```python
from build123d import *

# Parameters (mm, degrees)
SKETCH1_R           = 15.875
BOSS_EXTRUDE1_DEPTH = 76.2
SKETCH2_R           = 22.225
BOSS_EXTRUDE2_DEPTH = 152.4
SKETCH3_R           = 15.875
BOSS_EXTRUDE3_DEPTH = 76.2
FILLET1_R           = 0.254
FILLET2_R           = 0.254
FILLET3_R           = 0.254
FILLET4_R           = 0.254


with BuildPart() as part:
    # Sketch1 → Boss-Extrude1 (new body)
    with BuildSketch(Plane(origin=(0, 0, 0), x_dir=(1, 0, 0), z_dir=(0, 1, 0))):
        with Locations(Location((0, 0, 0), (0, 0, 90))):
            Circle(SKETCH1_R)
    extrude(amount=BOSS_EXTRUDE1_DEPTH)

    # Sketch2 → Boss-Extrude2 (add)
    with BuildSketch(Plane(origin=(0, 76.2, 0), x_dir=(1, 0, 0), z_dir=(0, 1, 0))):
        with Locations(Location((0, 0, 0), (0, 0, 90))):
            Circle(SKETCH2_R)
    extrude(amount=BOSS_EXTRUDE2_DEPTH)

    # Sketch3 → Boss-Extrude3 (add)
    with BuildSketch(Plane(origin=(0, 228.6, 0), x_dir=(1, 0, 0), z_dir=(0, 1, 0))):
        with Locations(Location((0, 0, 0), (0, 0, 90))):
            Circle(SKETCH3_R)
    extrude(amount=BOSS_EXTRUDE3_DEPTH)

    # Fillet1
    fillet1_edges = [part.edges().sort_by_distance(p)[0] for p in [
        (0, 76.2, 15.875),
    ]]
    fillet(fillet1_edges, radius=FILLET1_R)

    # Fillet2
    fillet2_edges = [part.edges().sort_by_distance(p)[0] for p in [
        (0, 228.6, 15.875),
    ]]
    fillet(fillet2_edges, radius=FILLET2_R)

    # Fillet3
    fillet3_edges = [part.edges().sort_by_distance(p)[0] for p in [
        (0, 228.6, 22.225),
    ]]
    fillet(fillet3_edges, radius=FILLET3_R)

    # Fillet4
    fillet4_edges = [part.edges().sort_by_distance(p)[0] for p in [
        (0, 76.2, 22.225),
    ]]
    fillet(fillet4_edges, radius=FILLET4_R)


solid = part.part
```
For this review, take the finished solid that the model builds, in its own axes (mm). A direction names the side the tool comes from. Coordinates: 2 decimals unless noted, no trailing zeros. Write each loop counter-clockwise with the first axis right and the second up, starting at its lowest first coordinate (ties: lowest second). Pieces come first, ordered by that corner, then holes. Notation, with made-up numbers: (-28, -6.5) - (-18, -6.5) arc R22 ccw to (-18, 9.5) - close; hole circle Ø2 at (36.5, 55). An arc over 180 degrees is marked (long way). Answer in a Markdown table with one row per item. Add a question column.
Q1. For probe 1 along Y at (x, z) = (-19, 1.5); probe 2 along Z at (x, y) = (-1.5, 173); probe 3 along Z at (x, y) = (19, 195), list the stretches that pass through material, from the lowest coordinate up.
Q2. We need section A-A, the plane z = 0. State the section outline as (x, y) points (3 decimals).
Q3. We need section D-D, the plane y = 133.5. State the section outline as (x, z) points (3 decimals), and give its area (3 significant figures).
Q4. Tool access review of faces 1 (the cylindrical face through (-18.74, 151.34, -11.95)), 2 (the cylindrical face through (15.497, 266.295, 3.441)), 3 (the cylindrical face through (15.497, 37.441, 3.441)): name each direction out of +Z, -Z, +X, -X, +Y, -Y from which nothing blocks a thin tool from reaching the whole face with its end or side.
Q5. We need section B-B, the plane x = 0. State the section outline as (y, z) points (3 decimals), and give its area (3 significant figures).
Q6. We need section C-C, the plane y = 233.5. State the section outline as (x, z) points (3 decimals), and give its area (3 significant figures).
Q7. For P1, Ø10, axis at x = 5.5, y = 123.5, coming from the -Z side; P2, Ø2, axis at y = 71, z = 2, coming from the +X side; P3, Ø3, axis at x = 6, y = 178.5, coming from the +Z side, all flat-tipped, find the tip position at first contact; note any pin that passes through.
Answer list:
| question | item | result |
|---|---|---|
| 1 | probe 1 | y = 76.2 to 228.6 |
| 1 | probe 2 | z = -22.17 to 22.17 |
| 1 | probe 3 | z = -11.53 to 11.53 |
| 2 | outline | (-22.225, 76.454) arc R0.254 ccw to (-21.971, 76.2) - (-16.129, 76.2) arc R0.254 cw to (-15.875, 75.946) - (-15.875, 0) - (15.875, 0) - (15.875, 75.946) arc R0.254 cw to (16.129, 76.2) - (21.971, 76.2) arc R0.254 ccw to (22.225, 76.454) - (22.225, 228.346) arc R0.254 ccw to (21.971, 228.6) - (16.129, 228.6) arc R0.254 cw to (15.875, 228.854) - (15.875, 304.8) - (-15.875, 304.8) - (-15.875, 228.854) arc R0.254 cw to (-16.129, 228.6) - (-21.971, 228.6) arc R0.254 ccw to (-22.225, 228.346) - close |
| 3 | outline | circle Ø44.45 at (0, 0) |
| 3 | area | 1,550 mm2 |
| 4 | face 1 | +Y, -Y |
| 4 | face 2 | +Y |
| 4 | face 3 | -Y |
| 5 | outline | (0, -15.875) - (75.946, -15.875) arc R0.254 cw to (76.2, -16.129) - (76.2, -21.971) arc R0.254 ccw to (76.454, -22.225) - (228.346, -22.225) arc R0.254 ccw to (228.6, -21.971) - (228.6, -16.129) arc R0.254 cw to (228.854, -15.875) - (304.8, -15.875) - (304.8, 15.875) - (228.854, 15.875) arc R0.254 cw to (228.6, 16.129) - (228.6, 21.971) arc R0.254 ccw to (228.346, 22.225) - (76.454, 22.225) arc R0.254 ccw to (76.2, 21.971) - (76.2, 16.129) arc R0.254 cw to (75.946, 15.875) - (0, 15.875) - close |
| 5 | area | 11,600 mm2 |
| 6 | outline | circle Ø31.75 at (0, 0) |
| 6 | area | 792 mm2 |
| 7 | P1 | stops at z = -22.22 |
| 7 | P2 | stops at x = 15.84 |
| 7 | P3 | stops at z = 21.76 |
